Geometry: final body of the model. Coordinates: model frame, mm. A direction names the side the tool comes from. Coordinates: 2 decimals unless noted, no trailing zeros. Write each loop counter-clockwise with the first axis right and the second up, starting at its lowest first coordinate (ties: lowest second). Pieces come first, ordered by that corner, then holes. Notation, with made-up numbers: (88, 86.25) - (122, 86.25) arc R15 cw to (122, 113.25) - close; hole circle Ø3 at (15.5, 73). An arc over 180 degrees is marked (long way). Answer as a JSON object with one key per item and string values. Group by question number.
Item 1: Section C-C on z = 29.5. Return loops of the section in (x, y), and give its area (3 significant figures).
Item 2: Section A-A on x = 0. State how many separate pieces and enclosed holes the cut face has, and give its area (3 significant figures).
Item 3: First-contact query: pin 1 Ø8 at (x, y) = (0, 0) entering from +Z; pin 2 Ø2 at (x, y) = (0, -7) entering from -Z; pin 3 Ø2 at (x, y) = (6, 0) entering from +Z; pin 4 Ø5 at (y, z) = (-3, 36.5) entering from -X. Flat tips, straight axial feed; report the tip coordinate or a pass-through.
Item 4: Section D-D on x = -7.25. Return loops of the section in (y, z).
Item 5: Section B-B on y = 2.25. Return loops of the section in (x, z).
Item 6: Set-up query: faces 5 (the flat face through (0, 3.377, 1)), 6 (the flat face through (-1, -6, 49)), 7 (the flat face through (6, 1, 49)). Return all of +Z, -Z, +X, -X, +Y, -Y with unobstructed straight access to the full face (end or side cutting, diameter ignored); none if empty.
Item 7: Line query: line 1 along Y through (x, z) = (0, 53.5); line 2 along Y through (x, z) = (-2.25, 21); line 3 along X through (y, z) = (-0.5, 48). Output: solid intervals per line, ascending. Write a range as from..to.
Item 8: Mould query, pull axis Z, two halves, no side actions, for faces 1 (the flat face through (0.1, 3.5, 47.353)), 2 (the flat face through (0, 6, 50.35)), 3 (the flat face through (0, -3.377, 1)), 4 (the flat face through (0, -6, 47.35)). Classes: pulls with the +Z half, pulls with the -Z half, needs draft (parallel to the pull), parting line crosses it, or undercut.
```python
from build123d import *

# Parameters (mm, degrees)
SKETCH050_R     = 3
PAD038_DEPTH    = 2
SKETCH051_R     = 4
SKETCH051_R_2   = 3
PAD039_DEPTH    = 45.35
PAD040_DEPTH    = 3
SKETCH053_R     = 4
SKETCH053_R_2   = 3
PAD041_DEPTH    = 20
SKETCH054_W     = 15
SKETCH054_H     = 3
POCKET_DEPTH    = 5
SKETCH055_R     = 3
POCKET001_DEPTH = 67.351


with BuildPart() as part:
    # Sketch050 → Pad038 (new body)
    with BuildSketch(Plane.XY):
        Polygon((1.95, 3.377499), (-1.95, 3.377499), (-3.9, 0), (-1.95, -3.377499), (1.95, -3.377499), (3.9, 0), align=None)
        Circle(SKETCH050_R, mode=Mode.SUBTRACT)
    extrude(amount=PAD038_DEPTH)

    # Sketch051 (on Face9 of Pad038) → Pad039 (join)
    with BuildSketch(Plane.XY.offset(2)):
        Circle(SKETCH051_R)
        Circle(SKETCH051_R_2, mode=Mode.SUBTRACT)
    extrude(amount=PAD039_DEPTH)

    # Sketch052 (on Face12 of Pad039) → Pad040 (join)
    with BuildSketch(Plane.XY.offset(47.35)):
        with BuildLine():
            Line((1, -8.798354), (1, -1))
            Line((1, -1), (9.477389, -1))
            ThreePointArc((9.477389, -1), (9.53, 0), (9.477389, 1))
            Line((9.477389, 1), (1, 1))
            Line((1, 1), (1, 8.798354))
            ThreePointArc((1, 8.798354), (0, 8.855), (-1, 8.798354))
            Line((-1, 8.798354), (-1, 1))
            Line((-1, 1), (-9.477389, 1))
            ThreePointArc((-9.477389, 1), (-9.53, 0), (-9.477389, -1))
            Line((-9.477389, -1), (-1, -1))
            Line((-1, -1), (-1, -8.798354))
            ThreePointArc((-1, -8.798354), (0, -8.855), (1, -8.798354))
        make_face()
    extrude(amount=PAD040_DEPTH)

    # Sketch053 (on Face19 of Pad040) → Pad041 (join)
    with BuildSketch(Plane.XY.offset(47.35)):
        Circle(SKETCH053_R)
        Circle(SKETCH053_R_2, mode=Mode.SUBTRACT)
    extrude(amount=PAD041_DEPTH)

    # Sketch054 (on Face26 of Pad041) → Pocket (cut)
    with BuildSketch(Plane(origin=(0, 1, 0), x_dir=(-1, 0, 0), z_dir=(0, 1, 0))):
        with Locations((0, 45.852941)):
            Rectangle(SKETCH054_W, SKETCH054_H)
    extrude(amount=POCKET_DEPTH, mode=Mode.SUBTRACT)

    # Sketch055 (on Face36 of Pocket) → Pocket001 (cut, through all)
    with BuildSketch(Plane.XY.offset(67.35)):
        Circle(SKETCH055_R)
    extrude(amount=-POCKET001_DEPTH, mode=Mode.SUBTRACT)


solid = part.part
```
Checks:
{
 "1": {"outline": "circle Ø8 at (0, 0); hole circle Ø6 at (0, 0)", "area": "22.0 mm^2"},
 "2": {"separate pieces": "3", "enclosed holes": "0", "area": "158 mm^2"},
 "3": {"pin 1": "z = 67.35", "pin 2": "z = 47.35", "pin 3": "z = 50.35", "pin 4": "x = -3.97"},
 "4": {"outline": "(-1, 47.35) - (1, 47.35) - (1, 50.35) - (-1, 50.35) - close"},
 "5": {"outline": "(-3.31, 2) - (-2.6, 2) - (-2.6, 0) - (-1.98, 0) - (-1.98, 44.35) - (-3.31, 44.35) - close; (-3.31, 47.35) - (-1.98, 47.35) - (-1.98, 67.35) - (-3.31, 67.35) - close; (1.98, 0) - (2.6, 0) - (2.6, 2) - (3.31, 2) - (3.31, 44.35) - (1.98, 44.35) - close; (1.98, 47.35) - (3.31, 47.35) - (3.31, 67.35) - (1.98, 67.35) - close"},
 "6": {"face 5": "-Z, +X, -X, +Y", "face 6": "+Z, -Z, -X, -Y", "face 7": "+X, +Y"},
 "7": {"line 1": "-4..-3, 3..4", "line 2": "-3.31..-1.98, 1.98..3.31", "line 3": "-9.52..-2.96, 2.96..9.52"},
 "8": {"face 1": "undercut", "face 2": "pulls with the +Z half", "face 3": "needs draft", "face 4": "pulls with the -Z half"}
}
